Can you work these out from the model? Positions are in its coordinate system, mm. Face numbers are marked on the shaded views. Coordinates: 2 decimals unless noted, no trailing zeros.
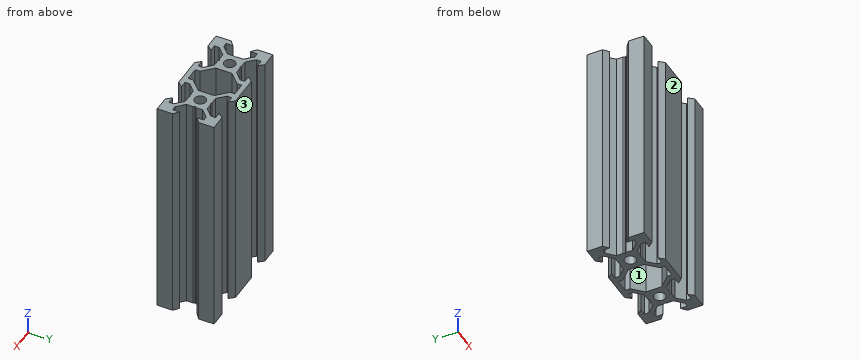
Autodesk Inventor part; units mm, degrees
ref_plane "YZ Plane" through (0, 0, 0) normal (1, 0, 0) x (0, 1, 0)
ref_plane "XZ Plane" through (0, 0, 0) normal (0, 1, 0) x (-1, 0, 0)
ref_plane "XY Plane" through (0, 0, 0) normal (0, 0, 1) x (1, 0, 0)
sketch "Sketch1" plane through (0, 0, 0) normal (0, 0, 1) x (1, 0, 0)
  line L0 (4.5, 8.2) -> (4.5, 6.5562)
  line L1 (6.9, 8.2) -> (4.5, 8.2)
  line L2 (5.3896, 10) -> (6.9, 8.2)
  line L3 (-5.3896, 10) -> (5.3896, 10)
  line L4 (-5.3896, 10) -> (-6.9, 8.2)
  line L5 (-6.9, 8.2) -> (-4.5, 8.2)
  line L6 (-4.5, 8.2) -> (-4.5, 6.5562)
  line L7 (-4.5, 6.5562) -> (-7.1607, 3.9)
  line L8 (-9.4804, 3.8998) -> (-7.1607, 3.9)
  line L9 (-9.4804, 3.8998) -> (-10, 3.5998)
  line L10 (-10.5196, 3.8998) -> (-10, 3.5998)
  line L11 (-12.8393, 3.9) -> (-10.5196, 3.8998)
  line L12 (-15.5, 6.5562) -> (-12.8393, 3.9)
  line L13 (-15.5, 8.2) -> (-15.5, 6.5562)
  line L14 (-13.1, 8.2) -> (-15.5, 8.2)
  line L15 (-14.6104, 10) -> (-13.1, 8.2)
  line L16 (-20, 10) -> (-14.6104, 10)
  line L17 (-20, 10) -> (-20, 4.6104)
  line L18 (-20, 4.6104) -> (-18.2, 3.1)
  line L19 (-18.2, 3.1) -> (-18.2, 5.5)
  line L20 (-16.5562, 5.5) -> (-18.2, 5.5)
  line L21 (-16.5562, 5.5) -> (-13.9, 2.8393)
  line L22 (-13.9, 0.5196) -> (-13.9, 2.8393)
  line L23 (-13.9, 0.5196) -> (-13.6, 0)
  line L24 (-13.6, 0) -> (-13.9, -0.5196)
  line L25 (-13.9, -2.8393) -> (-13.9, -0.5196)
  line L26 (-16.5562, -5.5) -> (-13.9, -2.8393)
  line L27 (-16.5562, -5.5) -> (-18.2, -5.5)
  line L28 (-18.2, -3.1) -> (-18.2, -5.5)
  line L29 (-20, -4.6104) -> (-18.2, -3.1)
  line L30 (-20, -10) -> (-20, -4.6104)
  line L31 (-20, -10) -> (-14.6104, -10)
  line L32 (-14.6104, -10) -> (-13.1, -8.2)
  line L33 (-13.1, -8.2) -> (-15.5, -8.2)
  line L34 (-15.5, -8.2) -> (-15.5, -6.5562)
  line L35 (-15.5, -6.5562) -> (-12.8393, -3.9)
  line L36 (-12.8393, -3.9) -> (-10.5196, -3.9002)
  line L37 (-10.5196, -3.9002) -> (-10, -3.6002)
  line L38 (-9.4804, -3.9002) -> (-10, -3.6002)
  line L39 (-9.4804, -3.9002) -> (-7.1604, -3.9002)
  line L40 (-4.5, -6.5562) -> (-7.1604, -3.9002)
  line L41 (-4.5, -8.2) -> (-4.5, -6.5562)
  line L42 (-6.9, -8.2) -> (-4.5, -8.2)
  line L43 (-5.3896, -10) -> (-6.9, -8.2)
  line L44 (-5.3896, -10) -> (5.3896, -10)
  line L45 (5.3896, -10) -> (6.9, -8.2)
  line L46 (6.9, -8.2) -> (4.5, -8.2)
  line L47 (4.5, -8.2) -> (4.5, -6.5562)
  line L48 (4.5, -6.5562) -> (7.1607, -3.9)
  line L49 (9.4808, -3.9) -> (7.1607, -3.9)
  line L50 (9.4808, -3.9) -> (10, -3.6002)
  line L51 (10.5192, -3.9) -> (10, -3.6002)
  line L52 (12.8393, -3.9) -> (10.5192, -3.9)
  line L53 (15.5, -6.5562) -> (12.8393, -3.9)
  line L54 (15.5, -8.2) -> (15.5, -6.5562)
  line L55 (13.1, -8.2) -> (15.5, -8.2)
  line L56 (14.6104, -10) -> (13.1, -8.2)
  line L57 (20, -10) -> (14.6104, -10)
  line L58 (20, -10) -> (20, -4.6104)
  line L59 (20, -4.6104) -> (18.2, -3.1)
  line L60 (18.2, -3.1) -> (18.2, -5.5)
  line L61 (16.5562, -5.5) -> (18.2, -5.5)
  line L62 (16.5562, -5.5) -> (13.9, -2.8393)
  line L63 (13.9, -2.8393) -> (13.9, -0.5196)
  line L64 (13.6, 0) -> (13.9, -0.5196)
  line L65 (13.9, 0.5196) -> (13.6, 0)
  line L66 (13.9, 0.5196) -> (13.9, 2.8393)
  line L67 (16.5562, 5.5) -> (13.9, 2.8393)
  line L68 (16.5562, 5.5) -> (18.2, 5.5)
  line L69 (18.2, 3.1) -> (18.2, 5.5)
  line L70 (20, 4.6104) -> (18.2, 3.1)
  line L71 (20, 10) -> (20, 4.6104)
  line L72 (20, 10) -> (14.6104, 10)
  line L73 (14.6104, 10) -> (13.1, 8.2)
  line L74 (13.1, 8.2) -> (15.5, 8.2)
  line L75 (15.5, 8.2) -> (15.5, 6.5562)
  line L76 (15.5, 6.5562) -> (12.8481, 3.8998)
  line L77 (10.5196, 3.8998) -> (12.8481, 3.8998)
  line L78 (10.5196, 3.8998) -> (10, 3.5998)
  line L79 (9.4804, 3.8998) -> (10, 3.5998)
  line L80 (7.1519, 3.8998) -> (9.4804, 3.8998)
  line L81 (4.5, 6.5562) -> (7.1519, 3.8998)
  circle A0 centre (-10, 0) radius 2
  circle A1 centre (10, 0) radius 2
  line L82 (6.1, 2.8393) -> (2.3832, 6.5562)
  line L83 (6.1, 2.8393) -> (6.1, -2.8393)
  line L84 (6.1, -2.8393) -> (2.3769, -6.5562)
  line L85 (2.3769, -6.5562) -> (2.3769, -8.2)
  line L86 (-2.3769, -8.2) -> (2.3769, -8.2)
  line L87 (-2.3769, -6.5562) -> (-2.3769, -8.2)
  line L88 (-6.1, -2.8393) -> (-2.3769, -6.5562)
  line L89 (-6.1, 2.8393) -> (-6.1, -2.8393)
  line L90 (-6.1, 2.8393) -> (-2.3832, 6.5562)
  line L91 (-2.3832, 6.5562) -> (-2.3832, 8.2)
  line L92 (-2.3832, 8.2) -> (2.3832, 8.2)
  line L93 (2.3832, 6.5562) -> (2.3832, 8.2)
  point P0 (0, 0)
  point P1 (0, 0)
extrude "Extrusion1" add sketch "Sketch1" along normal mid plane 80
properties part number "vslot_2040_80mm"
1. If I drill on L1, parallel to X at y = 7, z = 29; L2, parallel to Y at x = 10, z = 8; L3, parallel to Y at x = 5, z = -14.5, over which ranges is the centre line in solid material (lowest first)?
2. We'd pull the mould along Y, two halves only. Please class the marked faces 1, 2 and 3: released by +Y, released by -Y, zero draft, split by the parting line, or undercut.
3. If we section it at A-A, the plane z = 31: Count the separate pieces of the cut face and the enclosed holes in it, plus the area to 3 significant figures.
4. I'm going to push flat-ended pins straight in: P1, Ø2.5, axis at y = 1.5, z = -17.5, coming from the +X side; P2, Ø2, axis at x = -13, z = 3, coming from the -Y side; P3, Ø1.2, axis at x = -12, z = 9, coming from the -Y side. Where does each tip first touch, or does it pass through?
Answers:
1. L1: x = -20 to -15.5, -4.5 to -2.38, 2.38 to 4.5, 15.5 to 20
1. L2: y = -3.6 to -2, 2 to 3.6
1. L3: y = -10 to -8.2, -6.06 to -3.94, 3.94 to 6.06, 8.2 to 10
2. face 1: undercut
2. face 2: released by -Y
2. face 3: released by +Y
3. separate pieces: 1
3. enclosed holes: 3
3. area: 301 mm2
4. P1: stops at x = 13.9
4. P2: stops at y = -9.27
4. P3: stops at y = -3.9
